Geometry check sheet. Reference: the model listing, model coordinates, mm. A direction names the side the tool comes from. Round coordinates to 2 decimals unless told otherwise and drop trailing zeros. Write each loop counter-clockwise with the first axis right and the second up, starting at its lowest first coordinate (ties: lowest second). Pieces come first, ordered by that corner, then holes. Notation, with made-up numbers: (-36, 29.5) -> (-31, 29.5) arc R9 ccw to (-31, 34.5) -> close; hole circle Ø1 at (58, 83.5). An arc over 180 degrees is marked (long way). Return JSON: item names as keys, results as strings. Group by question number.
from build123d import *

# Parameters (mm, degrees)
SKETCH_1_R                   = 1.35
EXTRUDE_1_DEPTH              = 4
EXTRUDE_2_DEPTH              = 11
CUT_EXTRUDE_1_DEPTH          = 10
CUT_EXTRUDE_2_DEPTH          = 3
SKETCH_6_R                   = 1.6
CUT_EXTRUDE_3_DEPTH          = 31.233967875
SKETCH_7_R                   = 0.15
CUT_EXTRUDE_4_DEPTH          = 34.399294341
CUT_EXTRUDE_5_DEPTH          = 34.399294341
CUT_EXTRUDE_6_DEPTH          = 34.399294341
HOLE_WIZARD_M3_3_D           = 3.2
HOLE_WIZARD_M3_3_CSINK_D     = 6.3
HOLE_WIZARD_M3_3_CSINK_ANGLE = 90
EXTRUDE_3_DEPTH              = 4
FILLET_1_R                   = 1
CHAMFER_1_SIZE               = 5
CUT_EXTRUDE_7_DEPTH          = 4


with BuildPart() as part:
    # 草图1 → 凸台-拉伸1 (new body)
    with BuildSketch(Plane(origin=(0, 0, 0), x_dir=(1, 0, 0), z_dir=(0, 1, 0))):
        Polygon((7.6, -3.1), (7.6, 3.1), (-7.6, 3.1), (-7.6, -3.1), (-24, -3.1), (-24, 3.1), (-11.6, 3.1), (-11.6, 3.975781599), (-20.322903997, 13.736347087), (-15.849126022, 17.734510495), (-6.345187525, 7.1), (6.345187525, 7.1), (15.849126022, 17.734510495), (20.322903997, 13.736347087), (11.6, 3.975781599), (11.6, 3.1), (24, 3.1), (24, -3.1), align=None)
        with Locations(Location((-21, 0, 0), (0, 0, 270))):
            Circle(SKETCH_1_R, mode=Mode.SUBTRACT)
        with Locations(Location((-16.086933305, 13.498539803, 0), (0, 0, 270))):
            Circle(SKETCH_1_R, mode=Mode.SUBTRACT)
        with Locations(Location((16.086933305, 13.498539803, 0), (0, 0, 270))):
            Circle(SKETCH_1_R, mode=Mode.SUBTRACT)
        with Locations(Location((21, 0, 0), (0, 0, 270))):
            Circle(SKETCH_1_R, mode=Mode.SUBTRACT)
    extrude(amount=EXTRUDE_1_DEPTH)

    # 草图3 → 凸台-拉伸2 (add)
    with BuildSketch(Plane(origin=(0, 4, 0), x_dir=(1, 0, 0), z_dir=(0, 1, 0))):
        Polygon((-6.345187525, 7.1), (6.345187525, 7.1), (11.850962614, 13.26073252), (14.087851602, 11.261650816), (10.36863261, 7.1), (11.6, 7.1), (11.6, 2), (18, 2), (18, -2), (7.6, -2), (7.6, 3.1), (-7.6, 3.1), (-7.6, -3.1), (-18, -3.1), (-18, -0.1), (-11.6, -0.1), (-11.6, 7.1), (-10.36863261, 7.1), (-14.087851602, 11.261650816), (-11.850962614, 13.26073252), align=None)
    extrude(amount=EXTRUDE_2_DEPTH)

    # 草图4 → 切除-拉伸1 (cut)
    with BuildSketch(Plane.XY.offset(3.1)):
        Polygon((-11.6, 15), (-18, 4), (-18, 15), align=None)
        Polygon((18, 4), (18, 15), (11.6, 15), align=None)
    extrude(amount=-CUT_EXTRUDE_1_DEPTH, mode=Mode.SUBTRACT)

    # 草图5 → 切除-拉伸2 (cut)
    with BuildSketch(Plane(origin=(0, 0, 0), x_dir=(-0.6663605679521429, 0, 0.745629662418615), z_dir=(-0.745629662418615, 0, -0.6663605679521429))):
        Polygon((-12.203218518, 15), (-17.784609691, 4), (-17.784609691, 15), align=None)
    cut_extrude_2 = extrude(amount=-CUT_EXTRUDE_2_DEPTH, mode=Mode.SUBTRACT)

    # 镜向2: 切除-拉伸2 across plane
    add(cut_extrude_2.mirror(Plane(origin=(0, 0, 0), x_dir=(0, 0, 1), z_dir=(1, 0, 0))), mode=Mode.SUBTRACT)

    # 草图6 → 切除-拉伸3 (cut, through all)
    with BuildSketch(Plane(origin=(0, 0, -7.1), x_dir=(-1, 0, 0), z_dir=(0, 0, -1))):
        with Locations((0, 11.5)):
            Circle(SKETCH_6_R)
        with Locations((0, 3.5)):
            Circle(SKETCH_6_R)
    extrude(amount=-CUT_EXTRUDE_3_DEPTH, mode=Mode.SUBTRACT)

    # 草图7 → 切除-拉伸4 (cut, through all)
    with BuildSketch(Plane(origin=(0, 15, 0), x_dir=(1, 0, 0), z_dir=(0, 1, 0))):
        with Locations((7.45, 3.1)):
            Circle(SKETCH_7_R)
    extrude(amount=-CUT_EXTRUDE_4_DEPTH, mode=Mode.SUBTRACT)

    # 草图8 → 切除-拉伸5 (cut, through all)
    with BuildSketch(Plane(origin=(0, 15, 0), x_dir=(1, 0, 0), z_dir=(0, 1, 0))):
        Polygon((-7.6, 24.734510495), (-31, 24.734510495), (-31, -10.1), (-7.6, -10.1), (-7.6, 3.1), (-7.6, 7.1), (-2.6, 7.1), (-2.6, 24.734510495), align=None)
    extrude(amount=-CUT_EXTRUDE_5_DEPTH, mode=Mode.SUBTRACT)

    # 镜向3: part across plane


with BuildPart() as part_1:
    add(part.part)
    add(part.part.mirror(Plane.XY))

    # 草图9 → 切除-拉伸6 (cut, through all)
    with BuildSketch(Plane(origin=(0, 15, 0), x_dir=(1, 0, 0), z_dir=(0, 1, 0))):
        Polygon((6.345187525, -7.1), (11.6, -7.1), (11.6, -3.975781599), (21.345187525, -3.975781599), (21.345187525, -18.975781599), (6.345187525, -18.975781599), align=None)
    extrude(amount=-CUT_EXTRUDE_6_DEPTH, mode=Mode.SUBTRACT)

    # M3 锥坑高头螺钉的锥形沉头孔3 (through all)
    with Locations(Plane(origin=(0, 11.5, 7.1), x_dir=(1, 0, 0), z_dir=(0, 0, 1))):
        with Locations((0, 0), (0, -8)):
            CounterSinkHole(HOLE_WIZARD_M3_3_D / 2, HOLE_WIZARD_M3_3_CSINK_D / 2, counter_sink_angle=HOLE_WIZARD_M3_3_CSINK_ANGLE)

    # 草图12 → 凸台-拉伸3 (add)
    with BuildSketch(Plane(origin=(0, 4, 0), x_dir=(1, 0, 0), z_dir=(0, 1, 0))):
        Polygon((11.6, 3.975781599), (20.322903997, 13.736347087), (24, 3.1), (11.6, 3.1), align=None)
    extrude(amount=-EXTRUDE_3_DEPTH)

    # 圆角1
    fillet_1_edges = [part_1.edges().sort_by_distance(p)[0] for p in [
        (-7.6, 7.5, -7.1),
        (11.6, 7.5, 7.1),
        (-7.6, 7.5, 7.1),
        (15.849126022, 2, -17.734510495),
        (24, 2, 3.1),
        (11.6, 9.5, -7.1),
    ]]
    fillet(fillet_1_edges, radius=FILLET_1_R)

    # 倒角1
    # the kernel refuses this chamfer: 5 mm, written as the material it adds along each edge
    with BuildSketch(Plane(origin=(-2.48978233, 4, -7.1), x_dir=(0, -0.02749587661058641, -0.9996219169112968), z_dir=(1, 0, 0))) as chamfer_1_piece_1_section:
        Polygon((CHAMFER_1_SIZE * 0.999621916911, CHAMFER_1_SIZE * 0.0274958766106), (-CHAMFER_1_SIZE * 0.0274958766106, CHAMFER_1_SIZE * 0.999621916911), (0, 0), align=None)
    chamfer_1_piece_1 = extrude(amount=13.08978233, mode=Mode.PRIVATE)
    chamfer_1_piece_1 = split(chamfer_1_piece_1, bisect_by=Plane(origin=(10.479473381, 6.457230488, -7.224026197), z_dir=(0.7456296624186146, 0, 0.6663605679521433)), keep=Keep.TOP, mode=Mode.PRIVATE)
    add(chamfer_1_piece_1)
    with BuildSketch(Plane(origin=(10.6, 4, -6.1), x_dir=(0, 0, -1), z_dir=(-1, 0, 0))) as chamfer_1_piece_2_section:
        Polygon((1 + CHAMFER_1_SIZE, 0), (1, -CHAMFER_1_SIZE), (1, 0), align=None)
    chamfer_1_piece_2 = revolve(axis=Axis((10.6, 4, -6.1), (0, -1, 0)), revolution_arc=90, mode=Mode.PRIVATE)
    chamfer_1_piece_2 = split(chamfer_1_piece_2, bisect_by=Plane(origin=(10.960493571, 6.207373744, -7.762267712), z_dir=(0.7456296624186146, 0, 0.6663605679521433)), keep=Keep.TOP, mode=Mode.PRIVATE)
    add(chamfer_1_piece_2)
    with BuildSketch(Plane(origin=(11.6, 4, -2), x_dir=(0.9996219169112968, -0.027495876610586396, 0), z_dir=(0, 0, -1))) as chamfer_1_piece_3:
        Polygon((CHAMFER_1_SIZE * 0.999621916911, -CHAMFER_1_SIZE * 0.0274958766106), (-CHAMFER_1_SIZE * 0.0274958766106, -CHAMFER_1_SIZE * 0.999621916911), (0, 0), align=None)
    extrude(amount=4.1)

    # 草图13 → 切除-拉伸7 (cut)
    with BuildSketch(Plane.XY.offset(7.1)):
        Polygon((11.6, 4.849742261), (8.8, 0), (11.6, 0), align=None)
    extrude(amount=-CUT_EXTRUDE_7_DEPTH, mode=Mode.SUBTRACT)


solid = part_1.part
1) Tool access check on faces 4 (the face through (12, 0, -3)), 5 (the face through (10.22, 2.46, 5.13)), 6 (the face through (14.1, 6.5, -4)), 7 (the face through (4, 15, -4)), 8 (the face through (0, 7, -7.1)). Record the directions out of +Z, -Z, +X, -X, +Y, -Y that give a thin tool (end or side, any length) a straight path to the whole face; none if there is none.
2) Sectioned sample at C-C on z = 4.5. Enter the section's corners in (x, y).
3) Go/stop test with flat-tipped pins: P1, Ø1, axis at y = 12.5, z = -2, coming from the -X side; P2, Ø3.5, axis at y = 13, z = -4.5, coming from the +X side; P3, Ø4, axis at x = 0.5, y = 7.5, coming from the -Z side; P4, Ø3, axis at x = 0, y = 3.5, coming from the -Z side. Record where each tip stops, or that it passes through.
4) Mould release check, pull along Z, two halves, no side actions. Record for faces 1 (the face through (2, 7, 7.1)), 2 (the face through (14.755, 9.577, 0.028)), 3 (the face through (7.6, 7, 0)): +Z half, -Z half, draft (parallel to the pull), parting line (faces both ways), or undercut.
5) Material ranges on probe 1 along Z at (x, y) = (-3.5, 6.75); probe 2 along X at (y, z) = (2.7, 0); probe 3 along X at (y, z) = (11.5, 4.35), recorded low to high. Write a range as [from, to].
6) Sectioned sample at A-A on z = 0. Enter the section's corners in (x, y), and give its area (3 significant figures).
7) Sectioned sample at D-D on y = 3.5. State how many separate pieces and enclosed holes the cut face has, and give its area (3 significant figures).
8) Sectioned sample at B-B on x = 0. Enter the section's corners in (y, z), and give its area (3 significant figures).
Evaluation:
{
 "1": {"face 4": "+Z, -Z, +X, -X, -Y", "face 5": "+Z, +X, -Y", "face 6": "+X, +Y", "face 7": "+Z, -Z, +X, -X, +Y", "face 8": "-Z, -X, +Y, -Y"},
 "2": {"outline": "(-7.6, 0) -> (8.8, 0) -> (11.6, 4.85) -> (11.6, 15) -> (-7.6, 15) -> close; hole circle Ø3.2 at (0, 3.5); hole circle Ø3.2 at (0, 11.5)"},
 "3": {"P1": "stops at x = 7.6", "P2": "stops at x = 11.6", "P3": "stops at z = -7.1", "P4": "passes through"},
 "4": {"face 1": "+Z half", "face 2": "draft", "face 3": "undercut"},
 "5": {"probe 1": "z = [-7.1, -3.1], [3.1, 7.1]", "probe 2": "x = [7.6, 19.65], [22.35, 24]", "probe 3": "x = [-7.6, -1.6], [1.6, 11.6]"},
 "6": {"outline": "(7.6, 0) -> (19.65, 0) -> (19.65, 4) -> (18, 4) -> (11.6, 15) -> (7.6, 15) -> close; (22.35, 0) -> (24, 0) -> (24, 4) -> (22.35, 4) -> close", "area": "134 mm2"},
 "7": {"separate pieces": "3", "enclosed holes": "2", "area": "355 mm2"},
 "8": {"outline": "(0, -7.1) -> (1.9, -7.1) -> (1.9, -3.1) -> (0, -3.1) -> close; (0, 3.1) -> (1.9, 3.1) -> (1.9, 5.55) -> (0.35, 7.1) -> (0, 7.1) -> close; (5.1, -7.1) -> (9.9, -7.1) -> (9.9, -3.1) -> (5.1, -3.1) -> close; (5.1, 3.1) -> (9.9, 3.1) -> (9.9, 5.55) -> (8.35, 7.1) -> (6.65, 7.1) -> (5.1, 5.55) -> close; (13.1, -7.1) -> (15, -7.1) -> (15, -3.1) -> (13.1, -3.1) -> close; (13.1, 3.1) -> (15, 3.1) -> (15, 7.1) -> (14.65, 7.1) -> (13.1, 5.55) -> close", "area": "64.0 mm2"}
}
